Here's how the part is built. I have some questions about the finished solid (model axes, mm). Coordinates: 2 decimals unless noted, no trailing zeros. Loops run counter-clockwise (first coordinate to the right, second up) from the corner with the lowest first, then second, coordinate; pieces in that order, holes last. Notation, with made-up numbers: (50.25, 49.25) - (98.25, 49.25) arc R13 ccw to (98.25, 57.25) - close; hole circle Ø9 at (27.25, 4.5). An arc over 180 degrees is marked (long way). Use a Markdown table: item, result.
```python
from build123d import *

# Parameters (mm, degrees)
F0_R     = 6.35
F0_R_2   = 3.302
F1_DEPTH = 5.4864
F2_SIZE  = 0.762
F3_SIZE  = 0.254


with BuildPart() as f1:
    # F0 (on Right) → F1 (new body)
    with BuildSketch(Plane.YZ):
        Circle(F0_R)
        Circle(F0_R_2, mode=Mode.SUBTRACT)
    extrude(amount=F1_DEPTH)

    # F2
    f2_edges = [f1.edges().sort_by_distance(p)[0] for p in [
        (5.4864, -3.302, 0),
        (0, -3.302, 0),
    ]]
    chamfer(f2_edges, length=F2_SIZE)

    # F3
    f3_edges = [f1.edges().sort_by_distance(p)[0] for p in [
        (0, -6.35, 0),
        (5.4864, -6.35, 0),
    ]]
    chamfer(f3_edges, length=F3_SIZE)


solid = f1.part
```
Q1. I want a section at A-A, the plane y = 0. Write out the boundary of the cut face in (x, z), then the cut area to 3 significant figures.
Check values:
| item | result |
|---|---|
| outline | (0, -6.1) - (0.25, -6.35) - (5.23, -6.35) - (5.49, -6.1) - (5.49, -4.06) - (4.72, -3.3) - (0.76, -3.3) - (0, -4.06) - close; (0, 4.06) - (0.76, 3.3) - (4.72, 3.3) - (5.49, 4.06) - (5.49, 6.1) - (5.23, 6.35) - (0.25, 6.35) - (0, 6.1) - close |
| area | 32.2 mm^2 |
Q2. If we mould it in two halves opening along Y, with no side actions, what happens to faces 1 (the face through (2.71, -1.38, -6.2)), 2 (the face through (2.72, 3.05, -1.26)), 3 (the face through (0, -1.4, -4))? For each: pulls with the +Y half, pulls with the -Y half, needs draft (parallel to the pull), parting line crosses it, or undercut.
Check values:
| item | result |
|---|---|
| face 1 | parting line crosses it |
| face 2 | undercut |
| face 3 | needs draft |
Q3. I want a section at C-C, the plane x = 2.35. Write out the boundary of the cut face in (y, z), then the cut area to 3 significant figures.
Check values:
| item | result |
|---|---|
| outline | circle Ø12.7 at (0, 0); hole circle Ø6.6 at (0, 0) |
| area | 92.4 mm^2 |
Q4. Will these pins go through, and if not, where does the flat tip stop? P1, Ø1.5, axis at y = 0, z = -4.5, coming from the -X side; P2, Ø3, axis at x = 2, z = 3.5, coming from the +Y side.
Check values:
| item | result |
|---|---|
| P1 | x = 0 |
| P2 | y = 6.03 |
Q5. Please list where these lines run through material, in increasing order: L1, parallel to Z at x = 3.55, y = 0; L2, parallel to Z at x = 0.9, y = 1.5; L3, parallel to Y at x = 2.7, z = 2.75. Write a range as from..to.
Check values:
| item | result |
|---|---|
| L1 | -6.35..-3.3, 3.3..6.35 |
| L2 | -6.17..-2.94, 2.94..6.17 |
| L3 | -5.72..-1.83, 1.83..5.72 |
